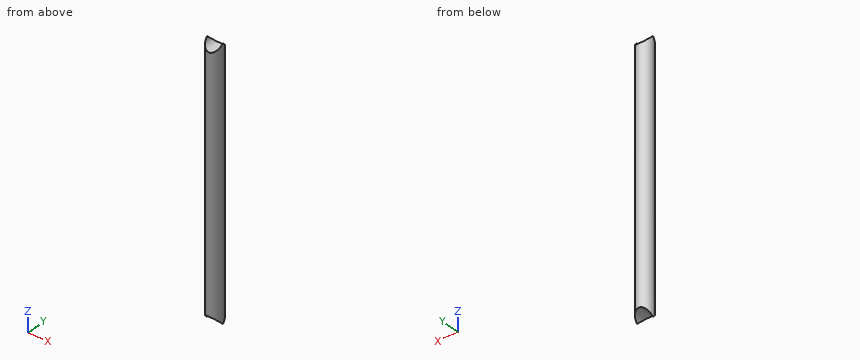
Autodesk Inventor part; units mm, degrees
ref_plane "Start plane" through (0, 0, 0) normal (0, 0, 1) x (1, 0, 0)
ref_plane "End plane" through (0, 0, 641.35) normal (0, 0, 1) x (1, 0, 0)
ref_plane "Work Plane4" through (0, 339.725, 660.4) normal (0, 0.7071, -0.7071) x (1, 0, 0)
ref_plane "Start plane" through (0, 0, 0) normal (0, 0, 1) x (1, 0, 0)
ref_plane "End plane" through (0, 0, 641.35) normal (0, 0, 1) x (1, 0, 0)
sketch "Sketch" plane through (0, 0, 0) normal (0, 0, 1) x (1, 0, 0)
  circle A0 centre (0, 0) radius 19.05
  dimension "d0" = 38.1
extrude "Body" add sketch "Sketch" along normal up to surface (641.35 mm away) from surface at 0
sketch "Sketch2" plane through (0, 0, 0) normal (0, 0, 1) x (1, 0, 0)
  line L0 (0, 0) -> (10, 0)
ref_plane "Work Plane3" through (0, 0, 0) normal (0, -1, 0) x (1, 0, 0)
sketch "Sketch3" plane through (0, 0, 0) normal (0, -1, 0) x (1, 0, 0)
  line L0 (-2, 0) -> (12, 0)
  line L1 (-2, 641.35) -> (12, 641.35)
  dimension "d7" = 641.35
ref_plane "Work Plane4" through (0, 339.725, 660.4) normal (0, 0.7071, -0.7071) x (1, 0, 0)
ref_plane "Work Plane5" through (0, -339.725, 660.4) normal (0, -0.7071, -0.7071) x (1, 0, 0)
ref_plane "Work Plane6" through (0, 0, 641.35) normal (0, -1, 0) x (1, 0, 0)
sketch "Sketch4" plane through (0, 0, 641.35) normal (0, -1, 0) x (1, 0, 0)
  circle A0 centre (0, 0) radius 19.05
extrude "Extrusion2" cut sketch "Sketch4" along normal up to surface from surface at -339.725 surface through (0, -339.725, 660.4) normal (0, -0.7071, -0.7071)
ref_plane "Work Plane7" through (0, -339.725, -19.05) normal (0, -0.7071, 0.7071) x (1, 0, 0)
ref_plane "Work Plane8" through (0, 339.725, -19.05) normal (0, 0.7071, 0.7071) x (1, 0, 0)
ref_plane "Work Plane9" through (0, 0, 0) normal (0, 1, 0) x (1, 0, 0)
sketch "Sketch5" plane through (0, 0, 0) normal (0, 1, 0) x (1, 0, 0)
  circle A0 centre (0, 0) radius 19.05
extrude "Extrusion3" cut sketch "Sketch5" along normal up to surface from surface at -339.725 surface through (0, 339.725, -19.05) normal (0, 0.7071, 0.7071)
equation "\"d0\" = Diam"
equation "\"d1\" = G_L"
equation "\"Diam\" = 38.1"
equation "\"G_L\" = d7"
equation "\"G_OFFSET_START\" = 0"
equation "\"G_OFFSET_END\" = 0"
equation "\"d5\" = G_OFFSET_END + B_L"
equation "\"B_L\" = 641.35"
properties part number "ANSI/AISC Rolled Steel - 1 1/2-25.25" material "Steel, Mild"
Geometry check sheet. Reference: the model listing, model coordinates, mm. Coordinates: 2 decimals unless noted, no trailing zeros. Loops run counter-clockwise (first coordinate to the right, second up) from the corner with the lowest first, then second, coordinate; pieces in that order, holes last.
Item 1: Go/stop test with flat-tipped pins: pin 1 Ø2 at (y, z) = (-10, 564) entering from -X; pin 2 Ø3 at (x, y) = (-1.5, -13.5) entering from +Z; pin 3 Ø10 at (x, y) = (-3.5, -10) entering from -Z. Record where each tip stops, or that it passes through.
Item 2: Sectioned sample at C-C, the plane x = 11. Record the boundary of the cut face in (y, z), then the cut area to 3 significant figures.
Item 3: Thickness scan on line 1 (Z direction, x = -0.5, y = -3.5); line 2 (Y direction, x = 2, z = 380.5). Record the ranges inside material, lowest first.
Item 4: Sectioned sample at B-B, the plane z = 420. Record the boundary of the cut face in (x, y).
Check result:
1. pin 1: stops at x = -16.79
1. pin 2: stops at z = 622.54
1. pin 3: stops at z = 17.05
2. outline: (-15.55, 15.55) - (15.55, 15.55) - (15.55, 625.8) - (-15.55, 625.8) - close
2. area: 19,000 mm2
3. line 1: z = 19.04 to 622.31
3. line 2: y = -18.94 to 18.94
4. outline: circle Ø38.1 at (0, 0)
